from build123d import *

# Parameters (mm, degrees)
SKETCH1_W           = 95.25
SKETCH1_H           = 107.95
BOSS_EXTRUDE1_DEPTH = 6.35
SKETCH2_W           = 31.75
SKETCH2_H           = 60.325
CUT_EXTRUDE1_DEPTH  = 7.35
SKETCH3_W           = 15.875
SKETCH3_H           = 6.35
SKETCH3_W_2         = 12.7
CUT_EXTRUDE2_DEPTH  = 7.35
SKETCH5_W           = 6.35
SKETCH5_H           = 12.7
CUT_EXTRUDE3_DEPTH  = 7.35
SKETCH6_W           = 6.35
SKETCH6_H           = 12.7
CUT_EXTRUDE4_DEPTH  = 7.35
LPATTERN1_COUNT     = 5
LPATTERN1_PITCH     = 25.4
FILLET1_R           = 6.35


with BuildPart() as part:
    # Sketch1 → Boss-Extrude1 (new body)
    with BuildSketch(Plane(origin=(0, 0, 0), x_dir=(0, 0, -1), z_dir=(1, 0, 0))):
        with Locations((47.625, 53.975)):
            Rectangle(SKETCH1_W, SKETCH1_H)
    extrude(amount=BOSS_EXTRUDE1_DEPTH)

    # Sketch2 → Cut-Extrude1 (cut, through all)
    with BuildSketch(Plane(origin=(6.35, 0, 0), x_dir=(0, 0, -1), z_dir=(1, 0, 0))):
        with Locations((73.025, 46.9875)):
            Rectangle(SKETCH2_W, SKETCH2_H)
    extrude(amount=-CUT_EXTRUDE1_DEPTH, mode=Mode.SUBTRACT)

    # Sketch3 → Cut-Extrude2 (cut, through all)
    with BuildSketch(Plane(origin=(6.35, 0, 0), x_dir=(0, 0, -1), z_dir=(1, 0, 0))):
        with Locations((7.9375, 104.775)):
            Rectangle(SKETCH3_W, SKETCH3_H)
        with Locations((34.925, 104.775)):
            Rectangle(SKETCH3_W_2, SKETCH3_H)
        with Locations((60.325, 104.775)):
            Rectangle(SKETCH3_W_2, SKETCH3_H)
        with Locations((87.3125, 104.775)):
            Rectangle(SKETCH3_W, SKETCH3_H)
    extrude(amount=-CUT_EXTRUDE2_DEPTH, mode=Mode.SUBTRACT)

    # Sketch5 → Cut-Extrude3 (cut, through all)
    with BuildSketch(Plane(origin=(6.35, 0, 0), x_dir=(0, 0, -1), z_dir=(1, 0, 0))):
        with Locations((92.075, 95.25)):
            Rectangle(SKETCH5_W, SKETCH5_H)
        with Locations((92.075, 6.35)):
            Rectangle(SKETCH5_W, SKETCH5_H)
    extrude(amount=-CUT_EXTRUDE3_DEPTH, mode=Mode.SUBTRACT)

    # Sketch6 → Cut-Extrude4 (cut, through all)
    with BuildSketch(Plane(origin=(6.35, 0, 0), x_dir=(0, 0, -1), z_dir=(1, 0, 0))):
        with Locations((3.175, 95.25)):
            Rectangle(SKETCH6_W, SKETCH6_H)
    cut_extrude4 = extrude(amount=-CUT_EXTRUDE4_DEPTH, mode=Mode.SUBTRACT)

    # LPattern1: Cut-Extrude4 ×5
    with Locations(*[(0, -i * LPATTERN1_PITCH, 0) for i in range(1, LPATTERN1_COUNT)]):
        add(cut_extrude4, mode=Mode.SUBTRACT)

    # Fillet1
    fillet1_edges = [part.edges().sort_by_distance(p)[0] for p in [
        (3.175, 16.825, -57.15),
        (3.175, 77.15, -57.15),
        (3.175, 77.15, -88.9),
        (3.175, 16.825, -88.9),
    ]]
    fillet(fillet1_edges, radius=FILLET1_R)


solid = part.part
Check sheet for the modelled part. Datum: model origin and axes. Units: mm. A direction names the side the tool comes from. Give positions to 0.01 mm unless a question says otherwise; leave off trailing zeros. Write each loop counter-clockwise with the first axis right and the second up, starting at its lowest first coordinate (ties: lowest second). Pieces come first, ordered by that corner, then holes. Notation, with made-up numbers: M -18.5,58.25 L 8.5,58.25 A32 cw 8.5,92.25 Z; hole C 71,62.25 d11. An arc over 180 degrees is marked long. Use one line per item in the form item = value.
(1) Section check A-A on y = 36. Record the boundary of the cut face in (x, z), plus the area to 3 significant figures.
Answer block:
outline = M 0,-95.25 L 6.35,-95.25 L 6.35,-88.9 L 0,-88.9 Z; M 0,-57.15 L 6.35,-57.15 L 6.35,0 L 0,0 Z
area = 403 mm2
(2) Tool access check on faces 1 (the flat face through (3, 70, -6.35)), 2 (the cylindrical face through (3.13, 75.24, -87.09)), 3 (the flat face through (3, 101.6, -60)), 4 (the flat face through (3, 95, -88.9)), 5 (the flat face through (3, 101.6, -11)). Record the directions out of +Z, -Z, +X, -X, +Y, -Y that give a thin tool (end or side, any length) a straight path to the whole face; none if there is none.
Answer block:
face_1 = +Z, +X, -X
face_2 = +X, -X
face_3 = +X, -X, +Y
face_4 = -Z, +X, -X, +Y
face_5 = +Z, +X, -X, +Y
(3) Section check D-D on y = 7.5. Record the boundary of the cut face in (x, z).
Answer block:
outline = M 0,-88.9 L 6.35,-88.9 L 6.35,0 L 0,0 Z
(4) Draft check along Y on faces 6 (the flat face through (3, 107.95, -73)), 7 (the flat face through (3, 95, -6.35)), 8 (the flat face through (3, 38.1, -3)). Enter one of: pulls with the +Y half, pulls with the -Y half, needs draft (parallel to the pull), parting line crosses it, or undercut.
Answer block:
face_6 = pulls with the +Y half
face_7 = needs draft
face_8 = undercut
(5) Section check B-B on z = -75. Record the boundary of the cut face in (x, y) (3 decimals), plus the area to 3 significant figures.
Answer block:
outline = M 0,0 L 6.35,0 L 6.35,16.825 L 0,16.825 Z; M 0,77.15 L 6.35,77.15 L 6.35,107.95 L 0,107.95 Z
area = 302 mm2
(6) Material ranges on line 1 along Y through (x, z) = (1, -5); line 2 along Z through (x, y) = (5, 58.5); line 3 along Z through (x, y) = (1.25, 66), recorded low to high.
Answer block:
line_1 = 0 to 12.7, 25.4 to 38.1, 50.8 to 63.5, 76.2 to 88.9
line_2 = -95.25 to -88.9, -57.15 to 0
line_3 = -95.25 to -88.9, -57.15 to -6.35
(7) Depth check by flat-ended pin: P1, Ø1.9, axis at x = 3.5, z = -90.5, coming from the -Y side; P2, Ø1.5, axis at x = 1.5, z = -82.5, coming from the +Y side; P3, Ø3, axis at x = 3.5, y = 105.5, coming from the -Z side (3 decimals). Enter the tip coordinate at first touch or a pass-through.
Answer block:
P1 = 12.7
P2 = 101.6
P3 = -79.375
(8) Section check C-C on z = -34.5. Record the boundary of the cut face in (x, y), plus the area to 3 significant figures.
Answer block:
outline = M 0,0 L 6.35,0 L 6.35,101.6 L 0,101.6 Z
area = 645 mm2
